```python
from build123d import *

# Parameters (mm, degrees)
CROQUIS1_W              = 320
CROQUIS1_H              = 320
SALIENTE_EXTRUIR2_DEPTH = 10
CROQUIS2_W              = 160
CROQUIS2_H              = 160
SALIENTE_EXTRUIR3_DEPTH = 58
CROQUIS3_R              = 19
CORTAR_EXTRUIR1_DEPTH   = 58
CROQUIS6_W              = 140
CROQUIS6_H              = 140
CROQUIS6_R              = 35
CORTAR_EXTRUIR5_DEPTH   = 60
CROQUIS7_W              = 20
CROQUIS7_H              = 10
CORTAR_EXTRUIR6_DEPTH   = 69


with BuildPart() as part:
    # Croquis1 → Saliente-Extruir2 (new body)
    with BuildSketch(Plane.XY):
        with Locations((-50, -50)):
            Rectangle(CROQUIS1_W, CROQUIS1_H)
    extrude(amount=SALIENTE_EXTRUIR2_DEPTH)

    # Croquis2 → Saliente-Extruir3 (add)
    with BuildSketch(Plane.XY):
        with Locations((-50, -50)):
            Rectangle(CROQUIS2_W, CROQUIS2_H)
    extrude(amount=-SALIENTE_EXTRUIR3_DEPTH)

    # Croquis3 → Cortar-Extruir1 (cut)
    with BuildSketch(Plane(origin=(0, 0, -58), x_dir=(-1, 0, 0), z_dir=(0, 0, -1))):
        with Locations((50, -50)):
            Circle(CROQUIS3_R)
    extrude(amount=-CORTAR_EXTRUIR1_DEPTH, mode=Mode.SUBTRACT)

    # Croquis6 → Cortar-Extruir5 (cut)
    with BuildSketch(Plane(origin=(0, 0, -58), x_dir=(-1, 0, 0), z_dir=(0, 0, -1))):
        with Locations((50, -50)):
            Rectangle(CROQUIS6_W, CROQUIS6_H)
        with Locations((50, -50)):
            Circle(CROQUIS6_R, mode=Mode.SUBTRACT)
    extrude(amount=-CORTAR_EXTRUIR5_DEPTH, mode=Mode.SUBTRACT)

    # Croquis7 → Cortar-Extruir6 (cut)
    with BuildSketch(Plane.XZ.offset(130)):
        with Locations((-50, -5)):
            Rectangle(CROQUIS7_W, CROQUIS7_H)
    extrude(amount=-CORTAR_EXTRUIR6_DEPTH, mode=Mode.SUBTRACT)


solid = part.part
```
Source: CAD feature listing. Evaluate the final solid. Frame: model axes, mm. A direction names the side the tool comes from. Give positions to 0.01 mm unless a question says otherwise; leave off trailing zeros. Loops run counter-clockwise (first coordinate to the right, second up) from the corner with the lowest first, then second, coordinate; pieces in that order, holes last. Notation, with made-up numbers: (-34.5, -20) - (11.5, -20) arc R23 cw to (11.5, 13) - close; hole circle Ø10 at (25, 13). An arc over 180 degrees is marked (long way). Use CSV: the item, a comma, the result in double quotes.
1) Cut plane A-A (z = -33). Output: boundary loops of the cut face in (x, y).
Worked out:
outline,"(-130, -130) - (30, -130) - (30, 30) - (-130, 30) - close; circle Ø70 at (-50, -50); hole (-120, -120) - (20, -120) - (20, 20) - (-120, 20) - close; hole circle Ø38 at (-50, -50)"
2) Cut plane D-D (x = -125). Output: boundary loops of the cut face in (y, z), and give its area (3 significant figures).
Worked out:
outline,"(-210, 0) - (-130, 0) - (-130, -58) - (30, -58) - (30, 0) - (110, 0) - (110, 10) - (-210, 10) - close"
area,"12,500 mm^2"
3) Set-up query: faces 4 (the flat face through (-51, 30, -29)), 5 (the flat face through (-40, -125, -5)), 6 (the flat face through (-49, 20, -28)), 7 (the flat face through (-52, 110, 5)), 8 (the flat face through (-50, -58, 0)). Return all of +Z, -Z, +X, -X, +Y, -Y with unobstructed straight access to the full face (end or side cutting, diameter ignored); none if empty.
Worked out:
face 4,"-Z, +X, -X, +Y"
face 5,"-Y"
face 6,"-Z"
face 7,"+Z, -Z, +X, -X, +Y"
face 8,"none"
4) Mould query, pull axis X, two halves, no side actions, for faces 1 (the flat face through (20, -51, -28)), 2 (the flat face through (30, -51, -29)), 3 (the flat face through (-52, -48, 10)). Classes: +X half, -X half, draft (parallel to the pull), parting line (faces both ways), or undercut.
Worked out:
face 1,"undercut"
face 2,"+X half"
face 3,"draft"
5) Cut plane B-B (x = -50). Output: boundary loops of the cut face in (y, z), and give its area (3 significant figures).
Worked out:
outline,"(-210, 0) - (-120, 0) - (-120, 2) - (-85, 2) - (-85, 0) - (-31, 0) - (-31, -58) - (-15, -58) - (-15, 2) - (20, 2) - (20, -58) - (30, -58) - (30, 0) - (110, 0) - (110, 10) - (-210, 10) - close; (-130, -58) - (-120, -58) - (-120, -10) - (-130, -10) - close; (-85, -58) - (-69, -58) - (-69, -10) - (-85, -10) - close"
area,"5,820 mm^2"
6) Line query: line 1 (X direction, y = -12, z = -11); line 2 (Y direction, x = -50, z = -35). Output: solid intervals per line, ascending.
Worked out:
line 1,"x = -130 to -120, 20 to 30"
line 2,"y = -130 to -120, -85 to -69, -31 to -15, 20 to 30"
7) Pin query (flat end, axial travel): P1, Ø12, axis at y = -93, z = -21, coming from the -X side; P2, Ø5, axis at x = -160.5, y = -74, coming from the -Z side; P3, Ø5, axis at y = -124, z = -7, coming from the +X side. Return the tip coordinate at first contact, or that it passes through.
Worked out:
P1,"stops at x = -130"
P2,"stops at z = 0"
P3,"stops at x = 30"
8) Cut plane C-C (y = -111.5). Output: boundary loops of the cut face in (x, z), and give its area (3 significant figures).
Worked out:
outline,"(-210, 0) - (-130, 0) - (-130, -58) - (-120, -58) - (-120, 2) - (20, 2) - (20, -58) - (30, -58) - (30, 0) - (110, 0) - (110, 10) - (-210, 10) - close"
area,"4,080 mm^2"
